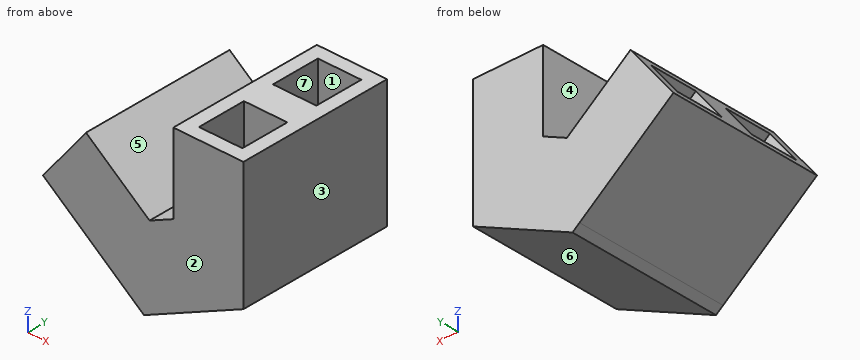
Autodesk Inventor part; units mm, degrees
ref_plane "Work Plane1" through (-0.53, 52.4069, -2.023) normal (-0.790155, 0, 0.6129071) x (0, 1, 0)
ref_plane "YZ Plane" through (0, 0, 0) normal (1, 0, 0) x (0, 1, 0)
ref_plane "XZ Plane" through (0, 0, 0) normal (0, 1, 0) x (-1, 0, 0)
sketch "Sketch1" plane through (0, 0, 0) normal (0, 0, 1) x (1, 0, 0)
  line L0 (19.1, 20.9) -> (4.5, 20.9) construction
  line L1 (19.1, 20.9) -> (19.1, 4.5) construction
  line L2 (19.1, 4.5) -> (4.5, 4.5) construction
  line L3 (4.5, 4.5) -> (4.5, 20.9) construction
  line L4 (4.5, 47.9069) -> (4.5, 31.5069) construction
  line L5 (19.1, 47.9069) -> (4.5, 47.9069) construction
  line L6 (19.1, 31.5069) -> (19.1, 47.9069) construction
  line L7 (4.5, 31.5069) -> (19.1, 31.5069) construction
  line L8 (0, 0) -> (0, 52.4069) construction
  line L9 (0, 0) -> (23.6, 0) construction
  line L10 (23.6, 0) -> (23.6, 52.4069) construction
  line L11 (0, 52.4069) -> (23.6, 52.4069) construction
  line L12 (0, 52.4069) -> (0, 0) construction
  line L13 (23.6, 0) -> (23.6, 52.4069) construction
  line L14 (0, 52.4069) -> (23.6, 52.4069)
  line L15 (23.6, 52.4069) -> (23.6, 0)
  line L16 (23.6, 0) -> (0, 0)
  line L17 (0, 0) -> (0, 52.4069)
  line L18 (4.5, 4.5) -> (4.5, 20.9) construction
  line L19 (19.1, 20.9) -> (19.1, 4.5) construction
  line L20 (4.5, 20.9) -> (19.1, 20.9)
  line L21 (19.1, 20.9) -> (19.1, 4.5)
  line L22 (19.1, 4.5) -> (4.5, 4.5)
  line L23 (4.5, 4.5) -> (4.5, 20.9)
  line L24 (4.5, 47.9069) -> (19.1, 47.9069)
  line L25 (19.1, 47.9069) -> (19.1, 31.5069)
  line L26 (19.1, 31.5069) -> (4.5, 31.5069)
  line L27 (4.5, 31.5069) -> (4.5, 47.9069)
  point P0 (0, 0)
  point P1 (-49.87, 37.7316)
extrude "Extrusion1" add sketch "Sketch1" along normal blind 40
sketch "Sketch2" plane through (0, 52.4069, 0) normal (0, 1, 0) x (1, 0, 0)
  line L0 (0, 0) -> (23.6, 0) construction
  line L1 (0, 0) -> (0, -40) construction
  line L2 (23.6, -40) -> (0, -40) construction
  line L3 (23.6, 0) -> (23.6, -40) construction
  line L4 (4.5, 0) -> (-0.53, 0)
  line L5 (4.5, 0) -> (9.53, 0) construction
  line L6 (-0.53, 0) -> (-0.53, 2.023)
  line L7 (-0.53, 0) -> (1.493, 0) construction
ref_plane "Work Plane1" through (-0.53, 52.4069, -2.023) normal (-0.790155, 0, 0.6129071) x (0, 1, 0)
sketch "Sketch3" plane through (-0.53, 52.4069, -2.023) normal (-0.790155, 0, 0.6129071) x (0, 1, 0)
  line L0 (-20.9, 14.6) -> (-20.9, 0) construction
  line L1 (-20.9, 14.6) -> (-4.5, 14.6) construction
  line L2 (-4.5, 14.6) -> (-4.5, 0) construction
  line L3 (-4.5, 0) -> (-20.9, 0) construction
  line L4 (-47.9069, 0) -> (-31.5069, 0) construction
  line L5 (-47.9069, 14.6) -> (-47.9069, 0) construction
  line L6 (-31.5069, 14.6) -> (-47.9069, 14.6) construction
  line L7 (-31.5069, 0) -> (-31.5069, 14.6) construction
  line L8 (0, -4.5) -> (-52.4069, -4.5) construction
  line L9 (0, -4.5) -> (0, 19.1) construction
  line L10 (0, 19.1) -> (-52.4069, 19.1) construction
  line L11 (-52.4069, -4.5) -> (-52.4069, 19.1) construction
  line L12 (-52.4069, -4.5) -> (0, -4.5) construction
  line L13 (0, 19.1) -> (-52.4069, 19.1) construction
  line L14 (-52.4069, -4.5) -> (-52.4069, 19.1)
  line L15 (-52.4069, 19.1) -> (0, 19.1)
  line L16 (0, 19.1) -> (0, -4.5)
  line L17 (0, -4.5) -> (-52.4069, -4.5)
  line L18 (-4.5, 0) -> (-20.9, 0) construction
  line L19 (-20.9, 14.6) -> (-4.5, 14.6) construction
  line L20 (-20.9, 0) -> (-20.9, 14.6)
  line L21 (-20.9, 14.6) -> (-4.5, 14.6)
  line L22 (-4.5, 14.6) -> (-4.5, 0)
  line L23 (-4.5, 0) -> (-20.9, 0)
  line L24 (-47.9069, 0) -> (-47.9069, 14.6)
  line L25 (-47.9069, 14.6) -> (-31.5069, 14.6)
  line L26 (-31.5069, 14.6) -> (-31.5069, 0)
  line L27 (-31.5069, 0) -> (-47.9069, 0)
  point P0 (-52.4069, -1.9233)
  point P1 (-49.87, 37.7316)
  point P2 (-4.5, 0)
extrude "Extrusion2" add sketch "Sketch3" along normal blind 40
sketch "Sketch4" plane through (0, 52.4069, 40) normal (0, 1, 0) x (1, 0, 0)
  line L0 (-12.2365, 57.115) -> (-43.8427, 32.5987) construction
  line L1 (1.0392, 40) -> (23.6, 40) construction
  line L2 (23.6, 40) -> (23.6, 43)
  line L3 (23.6, 40) -> (26.6, 40) construction
  line L4 (-12.2365, 57.115) -> (-9.8661, 58.9537)
  line L5 (-9.8661, 58.9537) -> (23.6, 43)
  line L6 (1.0392, 40) -> (-12.2365, 57.115) construction
  line L7 (-12.2365, 57.115) -> (1.0392, 40)
  line L8 (23.6, 40) -> (1.0392, 40) construction
  line L9 (1.0392, 40) -> (23.6, 40)
  point P0 (0, 40)
  point P1 (4.5, 40)
  point P2 (-0.53, 42.023)
  dimension "d9" = 3
  dimension "d10" = 90
  dimension "d11" = 3
extrude "Extrusion3" add sketch "Sketch4" against normal up to surface (52.4069 mm away)
sketch "Sketch5" plane through (0, 52.4069, 40) normal (0, 1, 0) x (1, 0, 0)
  line L0 (-9.8661, 58.9537) -> (23.6, 43) construction
  line L1 (0, 36.739) -> (0, 0) construction
  line L2 (0, 36.739) -> (0, 26.739)
  line L3 (0, 26.739) -> (-7.9847, 30.5454)
  line L4 (0, 36.739) -> (-7.9847, 30.5454)
  line L5 (0, 36.739) -> (-29.3781, 13.951) construction
  point P0 (0, 40)
extrude "Extrusion4" add sketch "Sketch5" against normal up to surface (52.4069 mm away)
properties part number "backwheel_Cap"
Verification items for the finished model (mm, model axes). Face numbers are marked on the shaded views. A direction names the side the tool comes from. Give positions to 0.01 mm unless a question says otherwise; leave off trailing zeros. Order: outer loops, then holes, each group sorted by start corner. A loop starts at its lowest first (then second) coordinate and runs counter-clockwise, first axis right, second up. Notation, with made-up numbers: (-30, 16.5) - (19, 16.5) arc R25 cw to (19, 30.5) - close; hole circle Ø4 at (88, 61.25). An arc over 180 degrees is marked (long way). Answer as CSV lines item,"result". Start each with the question number.
Item 1: Section check D-D, the plane z = 3. Record the boundary of the cut face in (x, y), plus the area to 3 significant figures.
Item 2: Access from +Z, -Z, +X, -X, +Y, -Y to the whole of each face (thin tool, end or side, straight path). Record for the marked faces 5, 6 and 7.
Item 3: Section check A-A, the plane z = 28. Record the boundary of the cut face in (x, y).
Item 4: Gauge pin test, flat ends, axial feed: pin 1 (12 mm diameter, centred on x = -2.5, y = 7.5, fed in from -Z); pin 2 (4 mm diameter, centred on y = 29.5, z = -6, fed in from -X); pin 3 (18 mm diameter, centred on x = -17, z = 3.5, fed in from -Y); pin 4 (5 mm diameter, centred on y = 26, z = -8, fed in from +X). Record the tip position at first contact, or that the pin passes through.
Item 5: Section check C-C, the plane x = -21. Record the boundary of the cut face in (y, z).
Item 6: Material ranges on L1, parallel to Y at x = -34, z = 11; L2, parallel to X at y = 44.5, z = 18; L3, parallel to X at y = 45.5, z = 30.5, recorded low to high.
Item 7: Mould release check, pull along X, two halves, no side actions. Record for the marked faces 1, 2, 3 and 4: released by +X, released by -X, zero draft, split by the parting line, or undercut.
Item 8: Section check B-B, the plane y = 22. Record the boundary of the cut face in (x, z), plus the area to 3 significant figures.
Filled in:
1,outline,"(-38.17, 0) - (23.6, 0) - (23.6, 52.41) - (-38.17, 52.41) - close; hole (-30.83, 4.5) - (-7.01, 4.5) - (-7.01, 20.9) - (-30.83, 20.9) - close; hole (-30.83, 31.51) - (-7.01, 31.51) - (-7.01, 47.91) - (-30.83, 47.91) - close; hole (4.5, 4.5) - (19.1, 4.5) - (19.1, 20.9) - (4.5, 20.9) - close; hole (4.5, 31.51) - (19.1, 31.51) - (19.1, 47.91) - (4.5, 47.91) - close"
1,area,"1,980 mm^2"
2,face 5,"+Z, +Y, -Y"
2,face 6,"-Z, +X, +Y, -Y"
2,face 7,"+Z"
3,outline,"(0, 0) - (23.6, 0) - (23.6, 52.41) - (0, 52.41) - close; hole (4.5, 4.5) - (19.1, 4.5) - (19.1, 20.9) - (4.5, 20.9) - close; hole (4.5, 31.51) - (19.1, 31.51) - (19.1, 47.91) - (4.5, 47.91) - close"
4,pin 1,"z = -18.3"
4,pin 2,"x = -29.14"
4,pin 3,"y = 0"
4,pin 4,"x = 18.36"
5,outline,"(0, -10.32) - (52.41, -10.32) - (52.41, 19.55) - (0, 19.55) - close; hole (4.5, -4.62) - (20.9, -4.62) - (20.9, 13.86) - (4.5, 13.86) - close; hole (31.51, -4.62) - (47.91, -4.62) - (47.91, 13.86) - (31.51, 13.86) - close"
6,L1,"0 to 4.5, 20.9 to 31.51, 47.91 to 52.41"
6,L2,"-26.34 to -19, 0 to 4.5, 19.1 to 23.6"
6,L3,"0 to 4.5, 19.1 to 23.6"
7,face 1,"undercut"
7,face 2,"zero draft"
7,face 3,"released by +X"
7,face 4,"undercut"
8,outline,"(-43.84, 7.4) - (-12.24, -17.11) - (-9.87, -18.95) - (23.6, -3) - (23.6, 40) - (0, 40) - (0, 13.26) - (-7.98, 9.45) - (-29.38, 26.05) - close"
8,area,"2,220 mm^2"
